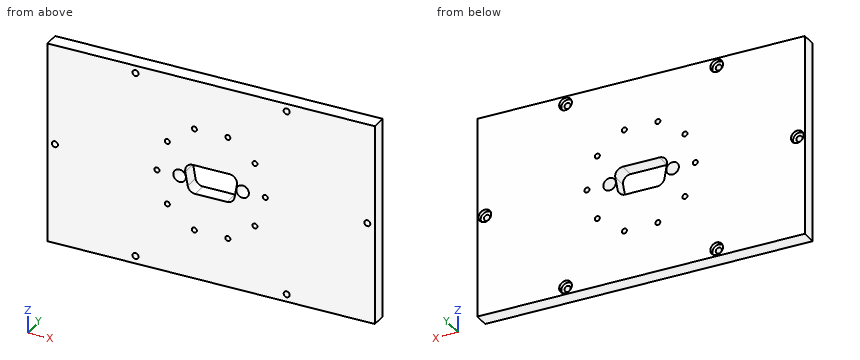
```python
from build123d import *

# Parameters (mm, degrees)
SKIZZE1_W                                    = 130
SKIZZE1_H                                    = 80
AUFSATZ_LINEAR_AUSTRAGEN1_DEPTH              = 6
F_2_4_2_4_DURCHMESSER_BOHRUNG1_D             = 2.4
F_2_4_2_4_DURCHMESSER_BOHRUNG1_DEPTH         = 10
F_2_4_2_4_DURCHMESSER_BOHRUNG1_CSINK_D       = 2.45
F_2_4_2_4_DURCHMESSER_BOHRUNG1_CSINK_ANGLE   = 90
F_2_4_2_4_DURCHMESSER_BOHRUNG1_TIP           = 0.721032743
STIRNSENKUNG_F_R_M2_FLACHKOPFSCHRAUB_2_COUNT = 2
STIRNSENKUNG_F_R_M2_FLACHKOPFSCHRAUB_2_PITCH = 48.918299235
STIRNSENKUNG_F_R_M2_FLACHKOPFSCHRAUB_3_COUNT = 2
STIRNSENKUNG_F_R_M2_FLACHKOPFSCHRAUB_3_PITCH = 74
STIRNSENKUNG_F_R_M2_FLACHKOPFSCHRAUB_4_COUNT = 2
STIRNSENKUNG_F_R_M2_FLACHKOPFSCHRAUB_4_PITCH = 95.268042911
STIRNSENKUNG_F_R_M2_FLACHKOPFSCHRAUB_5_COUNT = 2
STIRNSENKUNG_F_R_M2_FLACHKOPFSCHRAUB_5_PITCH = 99.161484458
STIRNSENKUNG_F_R_M2_FLACHKOPFSCHRAUB_6_COUNT = 2
STIRNSENKUNG_F_R_M2_FLACHKOPFSCHRAUB_6_PITCH = 60
SKIZZE8_R                                    = 1
SKIZZE8_R_2                                  = 2.5
SCHNITT_LINEAR_AUSTRAGEN1_DEPTH              = 6


with BuildPart() as part:
    # Skizze1 → Aufsatz-Linear austragen1 (new body)
    with BuildSketch(Plane(origin=(0, 0, 0), x_dir=(1, 0, 0), z_dir=(0, 1, 0))):
        with Locations((65, 40)):
            Rectangle(SKIZZE1_W, SKIZZE1_H)
    extrude(amount=AUFSATZ_LINEAR_AUSTRAGEN1_DEPTH)

    # Ø2.4 (2.4) Durchmesser Bohrung1
    with Locations(Plane(origin=(0, 6, 0), x_dir=(1, 0, 0), z_dir=(0, 1, 0))):
        with Locations((35, 77), (95, 77), (127, 40), (95, 3), (35, 3), (3, 40), (133.088689194, 32.803420387)):
            CounterSinkHole(F_2_4_2_4_DURCHMESSER_BOHRUNG1_D / 2, F_2_4_2_4_DURCHMESSER_BOHRUNG1_CSINK_D / 2, depth=F_2_4_2_4_DURCHMESSER_BOHRUNG1_DEPTH, counter_sink_angle=F_2_4_2_4_DURCHMESSER_BOHRUNG1_CSINK_ANGLE)
            with Locations((0, 0, -(F_2_4_2_4_DURCHMESSER_BOHRUNG1_DEPTH + F_2_4_2_4_DURCHMESSER_BOHRUNG1_TIP / 2))):  # 118° drill point
                Cone(0, F_2_4_2_4_DURCHMESSER_BOHRUNG1_D / 2, F_2_4_2_4_DURCHMESSER_BOHRUNG1_TIP, mode=Mode.SUBTRACT)

    # Skizze7 → Stirnsenkung für M2 Flachkopfschraube mit Schlitz1 (revolve, cut)
    with BuildSketch(Plane(origin=(95, 6, -3), x_dir=(0, 0, 1), z_dir=(1, 0, 0))):
        Polygon((0, 0), (0, 2.721032743), (1.2, 2), (1.2, 1.6), (2.5, 1.6), (2.5, 0.025), (2.525, 0), align=None)
    stirnsenkung_f_r_m2_flachkopfschraube_mi = revolve(axis=Axis((95, 12.35, -3), (0, -1, 0)), mode=Mode.SUBTRACT)

    # Stirnsenkung f_r M2 Flachkopfschraub 2: Stirnsenkung für M2 Flachkopfschraube mit Schlitz1 ×2
    with Locations(*[Vector(0.6541519329315842, 0, -0.7563631724521444) * (i * STIRNSENKUNG_F_R_M2_FLACHKOPFSCHRAUB_2_PITCH) for i in range(1, STIRNSENKUNG_F_R_M2_FLACHKOPFSCHRAUB_2_COUNT)]):
        add(stirnsenkung_f_r_m2_flachkopfschraube_mi, mode=Mode.SUBTRACT)

    # Stirnsenkung f_r M2 Flachkopfschraub 3: Stirnsenkung für M2 Flachkopfschraube mit Schlitz1 ×2
    with Locations(*[(0, 0, -i * STIRNSENKUNG_F_R_M2_FLACHKOPFSCHRAUB_3_PITCH) for i in range(1, STIRNSENKUNG_F_R_M2_FLACHKOPFSCHRAUB_3_COUNT)]):
        add(stirnsenkung_f_r_m2_flachkopfschraube_mi, mode=Mode.SUBTRACT)

    # Stirnsenkung f_r M2 Flachkopfschraub 4: Stirnsenkung für M2 Flachkopfschraube mit Schlitz1 ×2
    with Locations(*[Vector(-0.6298019584212194, 0, -0.7767557487195037) * (i * STIRNSENKUNG_F_R_M2_FLACHKOPFSCHRAUB_4_PITCH) for i in range(1, STIRNSENKUNG_F_R_M2_FLACHKOPFSCHRAUB_4_COUNT)]):
        add(stirnsenkung_f_r_m2_flachkopfschraube_mi, mode=Mode.SUBTRACT)

    # Stirnsenkung f_r M2 Flachkopfschraub 5: Stirnsenkung für M2 Flachkopfschraube mit Schlitz1 ×2
    with Locations(*[Vector(-0.9277795759357077, 0, -0.37312874249588235) * (i * STIRNSENKUNG_F_R_M2_FLACHKOPFSCHRAUB_5_PITCH) for i in range(1, STIRNSENKUNG_F_R_M2_FLACHKOPFSCHRAUB_5_COUNT)]):
        add(stirnsenkung_f_r_m2_flachkopfschraube_mi, mode=Mode.SUBTRACT)

    # Stirnsenkung f_r M2 Flachkopfschraub 6: Stirnsenkung für M2 Flachkopfschraube mit Schlitz1 ×2
    with Locations(*[(-i * STIRNSENKUNG_F_R_M2_FLACHKOPFSCHRAUB_6_PITCH, 0, 0) for i in range(1, STIRNSENKUNG_F_R_M2_FLACHKOPFSCHRAUB_6_COUNT)]):
        add(stirnsenkung_f_r_m2_flachkopfschraube_mi, mode=Mode.SUBTRACT)

    # Skizze8 → Schnitt-Linear austragen1 (cut)
    with BuildSketch(Plane(origin=(0, 6, 0), x_dir=(1, 0, 0), z_dir=(0, 1, 0))):
        with Locations(Location((47.606134621, 52.637382924, 0), (0, 0, 270))):
            Circle(SKIZZE8_R)
        with Locations(Location((58.356134621, 60.4477151, 0), (0, 0, 270))):
            Circle(SKIZZE8_R)
        with Locations(Location((71.643865379, 60.4477151, 0), (0, 0, 270))):
            Circle(SKIZZE8_R)
        with Locations(Location((82.393865379, 52.637382924, 0), (0, 0, 270))):
            Circle(SKIZZE8_R)
        with Locations(Location((86.5, 40, 0), (0, 0, 270))):
            Circle(SKIZZE8_R)
        with Locations(Location((82.393865379, 27.362617076, 0), (0, 0, 270))):
            Circle(SKIZZE8_R)
        with Locations(Location((71.643865379, 19.5522849, 0), (0, 0, 270))):
            Circle(SKIZZE8_R)
        with Locations(Location((58.356134621, 19.5522849, 0), (0, 0, 270))):
            Circle(SKIZZE8_R)
        with Locations(Location((47.606134621, 27.362617076, 0), (0, 0, 270))):
            Circle(SKIZZE8_R)
        with Locations(Location((43.5, 40, 0), (0, 0, 270))):
            Circle(SKIZZE8_R)
        with Locations(Location((77.5, 40, 0), (0, 0, 270))):
            Circle(SKIZZE8_R_2)
        with Locations(Location((52.5, 40, 0), (0, 0, 270))):
            Circle(SKIZZE8_R_2)
        with BuildLine():
            Line((72.295576741, 34.25), (57.704423259, 34.25))
            ThreePointArc((57.704423259, 34.25), (55.40628993, 35.321637171), (54.75, 37.770944533))
            Line((54.75, 37.770944533), (55.719798394, 43.270944533))
            ThreePointArc((55.719798394, 43.270944533), (56.745858824, 45.048133329), (58.674221653, 45.75))
            Line((58.674221653, 45.75), (71.325778347, 45.75))
            ThreePointArc((71.325778347, 45.75), (73.254141176, 45.048133329), (74.280201606, 43.270944533))
            Line((74.280201606, 43.270944533), (75.25, 37.770944533))
            ThreePointArc((75.25, 37.770944533), (74.59371007, 35.321637171), (72.295576741, 34.25))
        make_face()
    extrude(amount=-SCHNITT_LINEAR_AUSTRAGEN1_DEPTH, mode=Mode.SUBTRACT)


solid = part.part
```
The model under review builds one solid part; all positions refer to its coordinate system, in mm. Give positions to 0.01 mm unless a question says otherwise; leave off trailing zeros. Write each loop counter-clockwise with the first axis right and the second up, starting at its lowest first coordinate (ties: lowest second). Pieces come first, ordered by that corner, then holes. Notation, with made-up numbers: M -22,72 L 35,72 A11 ccw 35,93 Z; hole C 73,39.25 d11. An arc over 180 degrees is marked long. Write item = value, one per line. Start each with the question number.
Q1. We need section A-A (x = 52.5). State the section outline as (y, z) points, plus the area to 3 significant figures.
Q2. Clearance check with flat-ended pins moving along their axes: pin 1 (4.5 mm diameter, centred on x = 95, z = -3, fed in from +Y); pin 2 (5.5 mm diameter, centred on x = 34, z = -3.5, fed in from +Y). State where each tip first meets the part, or that it passes through.
Q3. For line 1 (X direction, y = 0.7, z = -42); line 2 (Z direction, x = 60, y = 1.3); line 3 (Z direction, x = 82, y = 1.55), list the stretches that pass through material, from the lowest coordinate up.
Result set:
q1.outline = M 0,-80 L 6,-80 L 6,-42.5 L 0,-42.5 Z; M 0,-37.5 L 6,-37.5 L 6,0 L 0,0 Z
q1.area = 450 mm2
q2.pin_1 = 4.4
q2.pin_2 = 6
q3.line_1 = 0 to 51, 54 to 55.5, 74.5 to 76, 79 to 130
q3.line_2 = -80 to -45.75, -34.25 to 0
q3.line_3 = -80 to -53.56, -51.72 to -28.28, -26.44 to 0
